from build123d import *

# Parameters (mm, degrees)
BOSS_EXTRUDE1_DEPTH = 10.05
BOSS_EXTRUDE2_DEPTH = 2.75
SKETCH3_R           = 7.5
BOSS_EXTRUDE3_DEPTH = 2.5
SKETCH4_R           = 6.75
BOSS_EXTRUDE4_DEPTH = 2
SKETCH5_R           = 5
BOSS_EXTRUDE5_DEPTH = 0.95
SKETCH6_R           = 3
SERVO_SPLINE_DEPTH  = 4
FILLET1_R           = 1
BOSS_EXTRUDE7_DEPTH = 0.35
CUT_EXTRUDE1_DEPTH  = 29.9
FILLET2_R           = 2
FILLET3_R           = 1
BOSS_EXTRUDE8_DEPTH = 5
BOSS_EXTRUDE8_TAPER = 7.5


with BuildPart() as part:
    # Sketch1 → Boss-Extrude1 (new body, symmetric)
    with BuildSketch(Plane(origin=(0, 0, 0), x_dir=(0, 0, -1), z_dir=(1, 0, 0))):
        Polygon((-20.05, 16.75), (20.05, 16.75), (20.05, 12.15), (26.5, 12.15), (26.5, 9.65), (20.05, 9.65), (20.05, -16.75), (-20.05, -16.75), (-20.05, 9.65), (-26.5, 9.65), (-26.5, 12.15), (-20.05, 12.15), align=None)
    extrude(amount=BOSS_EXTRUDE1_DEPTH, both=True)

    # Sketch2 → Boss-Extrude2 (add)
    with BuildSketch(Plane(origin=(0, 16.75, 0), x_dir=(1, 0, 0), z_dir=(0, 1, 0))):
        with BuildLine():
            Line((-8.875, 15.05), (8.875, 15.05))
            Line((8.875, 15.05), (8.875, -7.392918298))
            ThreePointArc((8.875, -7.392918298), (0, -19.25), (-8.875, -7.392918298))
            Line((-8.875, -7.392918298), (-8.875, 15.05))
        make_face()
    extrude(amount=BOSS_EXTRUDE2_DEPTH)

    # Sketch3 → Boss-Extrude3 (add)
    with BuildSketch(Plane(origin=(0, 16.75, 0), x_dir=(1, 0, 0), z_dir=(0, 1, 0))):
        with Locations((0, 10.05)):
            Circle(SKETCH3_R)
    extrude(amount=BOSS_EXTRUDE3_DEPTH)

    # Sketch4 → Boss-Extrude4 (add)
    with BuildSketch(Plane(origin=(0, 19.5, 0), x_dir=(1, 0, 0), z_dir=(0, 1, 0))):
        with Locations((0, -10)):
            Circle(SKETCH4_R)
    extrude(amount=BOSS_EXTRUDE4_DEPTH)

    # Sketch5 → Boss-Extrude5 (add)
    with BuildSketch(Plane(origin=(0, 21.5, 0), x_dir=(1, 0, 0), z_dir=(0, 1, 0))):
        with Locations((0, -10)):
            Circle(SKETCH5_R)
    extrude(amount=BOSS_EXTRUDE5_DEPTH)

    # Sketch6 → Servo Spline (add)
    with BuildSketch(Plane(origin=(0, 22.45, 0), x_dir=(1, 0, 0), z_dir=(0, 1, 0))):
        with Locations((0, -10)):
            Circle(SKETCH6_R)
    extrude(amount=SERVO_SPLINE_DEPTH)

    # Fillet1
    fillet1_edges = [part.edges().sort_by_distance(p)[0] for p in [
        (-8.875, 18.125, -15.05),
        (8.875, 18.125, -15.05),
    ]]
    fillet(fillet1_edges, radius=FILLET1_R)

    # Sketch7 → Boss-Extrude7 (add)
    with BuildSketch(Plane(origin=(0, 19.5, 0), x_dir=(1, 0, 0), z_dir=(0, 1, 0))):
        with BuildLine():
            Line((-7.875, 2.05), (-3, 2.05))
            Line((-3, 2.05), (-3, 1.55))
            ThreePointArc((-3, 1.55), (0, -1.45), (3, 1.55))
            Line((3, 1.55), (3, 2.05))
            Line((3, 2.05), (7.875, 2.05))
            ThreePointArc((7.875, 2.05), (8.582106781, 2.342893219), (8.875, 3.05))
            Line((8.875, 3.05), (8.875, 14.05))
            ThreePointArc((8.875, 14.05), (8.582106781, 14.757106781), (7.875, 15.05))
            Line((7.875, 15.05), (-7.875, 15.05))
            ThreePointArc((-7.875, 15.05), (-8.582106781, 14.757106781), (-8.875, 14.05))
            Line((-8.875, 14.05), (-8.875, 3.05))
            ThreePointArc((-8.875, 3.05), (-8.582106781, 2.342893219), (-7.875, 2.05))
        make_face()
    extrude(amount=BOSS_EXTRUDE7_DEPTH)

    # Sketch8 → Cut-Extrude1 (cut, through all)
    with BuildSketch(Plane(origin=(0, 12.15, 0), x_dir=(1, 0, 0), z_dir=(0, 1, 0))):
        with BuildLine():
            Line((6.730066226, -26.5), (3.169933774, -26.5))
            ThreePointArc((3.169933774, -26.5), (3.666925505, -26.154241731), (3.515549194, -25.568038035))
            ThreePointArc((3.515549194, -25.568038035), (4.95, -21.7), (6.384450806, -25.568038035))
            ThreePointArc((6.384450806, -25.568038035), (6.233074495, -26.154241731), (6.730066226, -26.5))
        make_face()
        with BuildLine():
            Line((-3.169933774, -26.5), (-6.730066226, -26.5))
            ThreePointArc((-6.730066226, -26.5), (-6.233074495, -26.154241731), (-6.384450806, -25.568038035))
            ThreePointArc((-6.384450806, -25.568038035), (-4.95, -21.7), (-3.515549194, -25.568038035))
            ThreePointArc((-3.515549194, -25.568038035), (-3.666925505, -26.154241731), (-3.169933774, -26.5))
        make_face()
        with BuildLine():
            Line((-6.730066226, 26.5), (-3.169933774, 26.5))
            ThreePointArc((-3.169933774, 26.5), (-3.666925505, 26.154241731), (-3.515549194, 25.568038035))
            ThreePointArc((-3.515549194, 25.568038035), (-4.95, 21.7), (-6.384450806, 25.568038035))
            ThreePointArc((-6.384450806, 25.568038035), (-6.233074495, 26.154241731), (-6.730066226, 26.5))
        make_face()
        with BuildLine():
            Line((3.169933774, 26.5), (6.730066226, 26.5))
            ThreePointArc((6.730066226, 26.5), (6.233074495, 26.154241731), (6.384450806, 25.568038035))
            ThreePointArc((6.384450806, 25.568038035), (4.95, 21.7), (3.515549194, 25.568038035))
            ThreePointArc((3.515549194, 25.568038035), (3.666925505, 26.154241731), (3.169933774, 26.5))
        make_face()
    extrude(amount=-CUT_EXTRUDE1_DEPTH, mode=Mode.SUBTRACT)

    # Fillet2
    fillet2_edges = [part.edges().sort_by_distance(p)[0] for p in [
        (10.05, 10.9, 26.5),
        (-10.05, 10.9, -26.5),
        (-10.05, 10.9, 26.5),
        (10.05, 10.9, -26.5),
    ]]
    fillet(fillet2_edges, radius=FILLET2_R)

    # Fillet3
    fillet3_edges = [part.edges().sort_by_distance(p)[0] for p in [
        (-10.05, 14.45, -20.05),
        (-10.05, -3.55, -20.05),
        (-10.05, -3.55, 20.05),
        (-10.05, 14.45, 20.05),
        (10.05, -3.55, 20.05),
        (10.05, -3.55, -20.05),
        (10.05, 14.45, -20.05),
        (10.05, 14.45, 20.05),
    ]]
    fillet(fillet3_edges, radius=FILLET3_R)

    # Sketch9 → Boss-Extrude8 (add)
    with BuildSketch(Plane.XY.offset(20.05)):
        with BuildLine():
            Line((-2.5, -14.25), (2.5, -14.25))
            ThreePointArc((2.5, -14.25), (3.207106781, -13.957106781), (3.5, -13.25))
            Line((3.5, -13.25), (3.5, -10.75))
            ThreePointArc((3.5, -10.75), (3.207106781, -10.042893219), (2.5, -9.75))
            Line((2.5, -9.75), (-2.5, -9.75))
            ThreePointArc((-2.5, -9.75), (-3.207106781, -10.042893219), (-3.5, -10.75))
            Line((-3.5, -10.75), (-3.5, -13.25))
            ThreePointArc((-3.5, -13.25), (-3.207106781, -13.957106781), (-2.5, -14.25))
        make_face()
    extrude(amount=BOSS_EXTRUDE8_DEPTH, taper=BOSS_EXTRUDE8_TAPER)


solid = part.part
Check sheet for the modelled part. Datum: model origin and axes. Units: mm. A direction names the side the tool comes from. Round coordinates to 2 decimals unless told otherwise and drop trailing zeros. Order: outer loops, then holes, each group sorted by start corner. A loop starts at its lowest first (then second) coordinate and runs counter-clockwise, first axis right, second up. Notation, with made-up numbers: M 88,10.5 L 123,10.5 A9 cw 123,22.5 Z; hole C 55.5,61.5 d6. An arc over 180 degrees is marked long. One line per item, written item: value. Start each with the question number.
1. Section check D-D on z = 23.9. Enter the section's corners in (x, y), and give its area (3 significant figures).
2. Release check for a two-part mould opening along Z. For faces 1 (the flat face through (-8.875, 18, -3)), 2 (the cylindrical face through (-4.9, 10.9, -21.7)), 3 (the flat face through (-7, 11, -26.5)) record: released by +Z, released by -Z, zero draft, split by the parting line, or undercut.
3. Section check C-C on z = -12.5. Enter the section's corners in (x, y) (3 decimals).
4. Access from +Z, -Z, +X, -X, +Y, -Y to the whole of each face (thin tool, end or side, straight path). Record for faces 4 (the flat face through (-0.035, -10.075, 22.515)), 5 (the cylindrical face through (0, 24, 7)), 6 (the flat face through (0.1, 19.7, -15.05)), 7 (the flat face through (0, -3, -20.05)), 8 (the flat face through (-10.05, 0, 0)).
5. Gauge pin test, flat ends, axial feed: P1, Ø1, axis at x = -7.5, z = 8, coming from the +Y side; P2, Ø3.5, axis at y = 17.5, z = -3, coming from the -X side; P3, Ø2, axis at x = -1.5, z = -16, coming from the +Y side; P4, Ø1.4, axis at x = -2, y = 15.5, coming from the +Z side. Record the tip position at first contact, or that the pin passes through.
6. Section check B-B on y = -11.5. Enter the section's corners in (x, z), and give its area (3 significant figures).
7. Scan lines: line 1 along X through (y, z) = (11.4, 23.9); line 2 along X through (y, z) = (10, 23); line 3 along Z through (x, y) = (-9, -7). Record each from-to range of solid material in increasing order.
8. Section check A-A on z = -23.9. Enter the section's corners in (x, y), and give its area (4 significant figures).
Results found:
1. outline: M -10.05,9.65 L -7.15,9.65 L -7.15,12.15 L -10.05,12.15 Z; M -2.99,-13.25 A0.49 ccw -2.5,-13.74 L 2.5,-13.74 A0.49 ccw 2.99,-13.25 L 2.99,-10.75 A0.49 ccw 2.5,-10.26 L -2.5,-10.26 A0.49 ccw -2.99,-10.75 Z; M -2.75,9.65 L 2.75,9.65 L 2.75,12.15 L -2.75,12.15 Z; M 7.15,9.65 L 10.05,9.65 L 10.05,12.15 L 7.15,12.15 Z
1. area: 48.9 mm^2
2. face 1: zero draft
2. face 2: undercut
2. face 3: released by -Z
3. outline: M -10.05,-16.75 L 10.05,-16.75 L 10.05,16.75 L 8.875,16.75 L 8.875,19.85 L -8.875,19.85 L -8.875,16.75 L -10.05,16.75 Z
4. face 4: +Z, +X, -X
4. face 5: +Y
4. face 6: -Z, +Y
4. face 7: -Z, +X, -X, -Y
4. face 8: +Z, -Z, -X, +Y, -Y
5. P1: y = 19.5
5. P2: x = -10.05
5. P3: y = 19.85
5. P4: z = 20.05
6. outline: M -10.05,-19.05 A1 ccw -9.05,-20.05 L 9.05,-20.05 A1 ccw 10.05,-19.05 L 10.05,19.05 A1 ccw 9.05,20.05 L 3.5,20.05 L 2.84,25.05 L -2.84,25.05 L -3.5,20.05 L -9.05,20.05 A1 ccw -10.05,19.05 Z
6. area: 837 mm^2
7. line 1: -10.05 to -7.15, -2.75 to 2.75, 7.15 to 10.05
7. line 2: -10.05 to -6.96, -2.94 to 2.94, 6.96 to 10.05
7. line 3: -20.05 to 20.05
8. outline: M -10.05,9.65 L -7.15,9.65 L -7.15,12.15 L -10.05,12.15 Z; M -2.75,9.65 L 2.75,9.65 L 2.75,12.15 L -2.75,12.15 Z; M 7.15,9.65 L 10.05,9.65 L 10.05,12.15 L 7.15,12.15 Z
8. area: 28.25 mm^2
